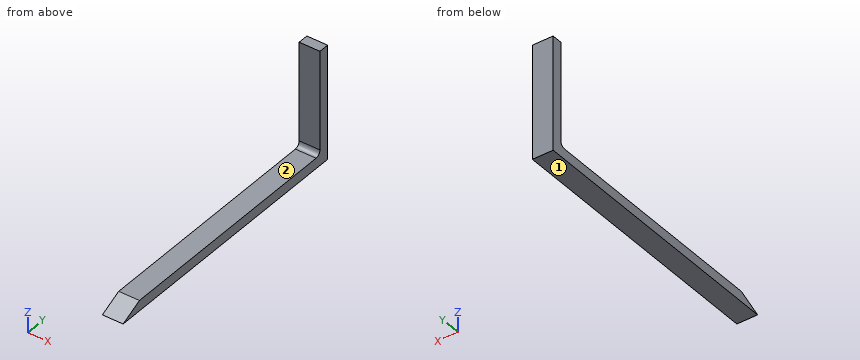
```python
from build123d import *

# Parameters (mm, degrees)
F1_DEPTH = 101.6
F2_R     = 25.4
F3_R     = 25.4
F4_DEPTH = 101.6
F5_ANGLE = 180


# Not quite as in the source:
# - a feature names something its author has since deleted; it is built from what else it names


with BuildPart() as f1:
    # F0 (on Right) → F1 (new body)
    with BuildSketch(Plane.YZ):
        Polygon((0, 38.1), (0, 0), (1352.55, 0), (1244.6, 50.8), (50.8, 50.8), (50.8, 558.8), (0, 558.8), align=None)
    extrude(amount=F1_DEPTH)

    # F2
    f2_edges = [f1.edges().sort_by_distance(p)[0] for p in [
        (50.8, 0, 0),
    ]]
    fillet(f2_edges, radius=F2_R)

    # F3
    f3_edges = [f1.edges().sort_by_distance(p)[0] for p in [
        (50.8, 50.8, 50.8),
    ]]
    fillet(f3_edges, radius=F3_R)

    # F0 (on Right) → F4 (join)
    with BuildSketch(Plane.YZ):
        Polygon((0, 38.1), (0, 0), (1352.55, 0), (1244.6, 50.8), (50.8, 50.8), (50.8, 558.8), (0, 558.8), align=None)
    extrude(amount=F4_DEPTH)


with BuildPart() as f1_1:
    # F5: moved
    add(f1.part.rotate(Axis((101.6, 0, 279.4), (0, 0, 1)), F5_ANGLE))


solid = f1_1.part
```
CAD build for the part. Positions are in the model's coordinates, mm. Face numbers are marked on the shaded views. A direction names the side the tool comes from. Round coordinates to 2 decimals unless told otherwise and drop trailing zeros. Order: outer loops, then holes, each group sorted by start corner. A loop starts at its lowest first (then second) coordinate and runs counter-clockwise, first axis right, second up.
Item 1: Tool access for the marked faces 1 and 2: list every direction of +Z, -Z, +X, -X, +Y, -Y with a clear straight run to the whole face (end or side of a thin tool).
Item 2: Saw through at A-A on x = 179. Write the cut outline in (y, z).
Item 3: Saw through at C-C on y = -850.5. Write the cut outline in (x, z), then the cut area to 3 significant figures.
Item 4: Pin check, flat tip, straight feed: pin 1 (1 mm diameter, centred on x = 144, y = -274, fed in from +Z). Stop position of the tip, or through.
Item 5: Probe line 1 along Z through (x, y) = (130.5, -934.5); line 2 along Y through (x, z) = (132, 93.5); line 3 along Y through (x, z) = (115, 33.5). List the from-to ranges inside material, lowest first.
Item 6: Saw through at B-B on z = 388.5. Write the cut outline in (x, y), then the cut area to 3 significant figures.
Reported:
1. face 1: -Z, +X, -X, +Y, -Y
1. face 2: +Z, +X, -X, -Y
2. outline: (-1352.55, 0) - (0, 0) - (0, 558.8) - (-50.8, 558.8) - (-50.8, 76.2) arc R25.4 cw to (-76.2, 50.8) - (-1244.6, 50.8) - close
3. outline: (101.6, 0) - (203.2, 0) - (203.2, 50.8) - (101.6, 50.8) - close
3. area: 5,160 mm2
4. pin 1: stops at z = 50.8
5. line 1: z = 0 to 50.8
5. line 2: y = -50.8 to 0
5. line 3: y = -1281.36 to 0
6. outline: (101.6, -50.8) - (203.2, -50.8) - (203.2, 0) - (101.6, 0) - close
6. area: 5,160 mm2
